Study the drawing (mm; zero at the part's minimum x, y, z) and answer. Round coordinates to 2 decimals unless told otherwise and drop trailing zeros. Order: outer loops, then holes, each group sorted by start corner. A loop starts at its lowest first (then second) coordinate and runs counter-clockwise, first axis right, second up. Notation, with made-up numbers: (76.5, -19.5) -> (101.5, -19.5) arc R15 cw to (101.5, 5.5) -> close; hole circle Ø4 at (16.5, 42.25). An arc over 180 degrees is marked (long way). Use one line per item in the form item = value.
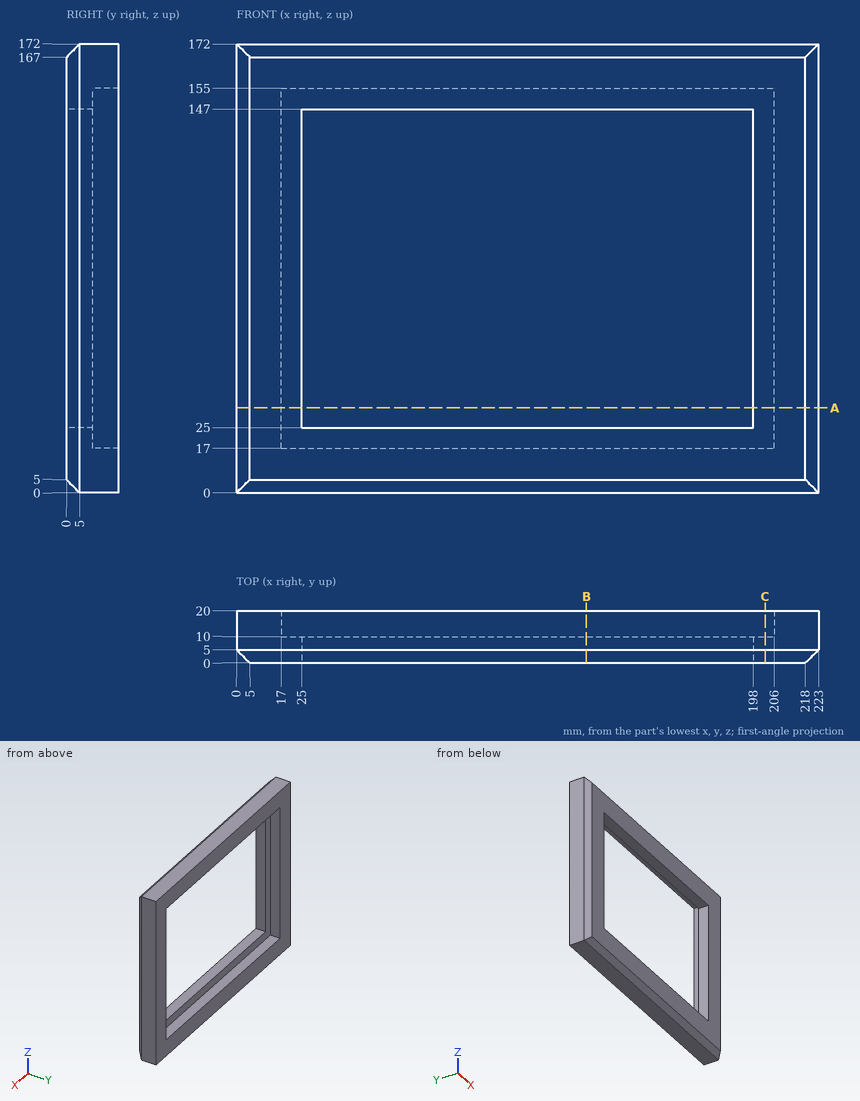
Item 1: Consider line 1 along Z through (x, y) = (194.5, 9.75); line 2 along Z through (x, y) = (77, 18.75); line 3 along X through (y, z) = (15, 34). Determine where each line is inside the solid, lowest interval first.
Findings:
line_1 = 0 to 25, 147 to 172
line_2 = 0 to 17, 155 to 172
line_3 = 0 to 17, 206 to 223
Item 2: The part is cut by section C-C, the plane x = 202.5. Give the vertices of the cut face in (y, z).
Findings:
outline = (0, 5) -> (5, 0) -> (20, 0) -> (20, 17) -> (10, 17) -> (10, 155) -> (20, 155) -> (20, 172) -> (5, 172) -> (0, 167) -> close
Item 3: The part is cut by section B-B, the plane x = 134. Give the vertices of the cut face in (y, z).
Findings:
outline = (0, 5) -> (5, 0) -> (20, 0) -> (20, 17) -> (10, 17) -> (10, 25) -> (0, 25) -> close; (0, 147) -> (10, 147) -> (10, 155) -> (20, 155) -> (20, 172) -> (5, 172) -> (0, 167) -> close
Item 4: The part is cut by section A-A, the plane z = 32.5. Give the vertices of the cut face in (x, y), and give its area (3 significant figures).
Findings:
outline = (0, 5) -> (5, 0) -> (25, 0) -> (25, 10) -> (17, 10) -> (17, 20) -> (0, 20) -> close; (198, 0) -> (218, 0) -> (223, 5) -> (223, 20) -> (206, 20) -> (206, 10) -> (198, 10) -> close
area = 815 mm^2
Item 5: Flat-ended cylindrical pins translate along their axes: P1, Ø5, axis at x = 198.5, z = 132.5, coming from the -Y side; P2, Ø1, axis at x = 26, z = 69.5, coming from the -Y side. Find the tip coordinate at first contact, or state that the pin passes through.
Findings:
P1 = 0
P2 = through
